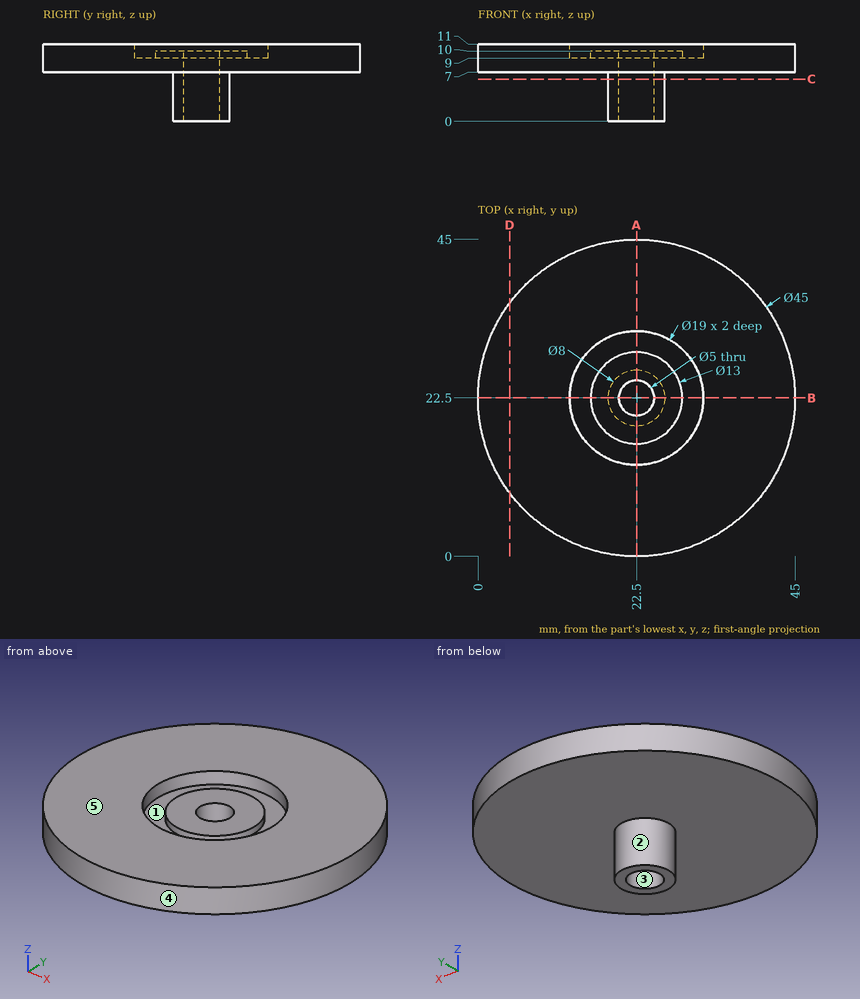
Check sheet for the drawn part. Datum: minimum x, y, z corner. Units: mm. A direction names the side the tool comes from. Give positions to 0.01 mm unless a question says otherwise; leave off trailing zeros. Order: outer loops, then holes, each group sorted by start corner. A loop starts at its lowest first (then second) coordinate and runs counter-clockwise, first axis right, second up. Notation, with made-up numbers: (5.5, 25) -> (40.5, 25) arc R22 cw to (40.5, 42) -> close; hole circle Ø4 at (-35.75, 85.25). An arc over 180 degrees is marked (long way). Use a Markdown table: item, result.
1) Mould release check, pull along X, two halves, no side actions. Record for the marked faces 3, 4 and 5: pulls with the +X half, pulls with the -X half, needs draft (parallel to the pull), parting line crosses it, or undercut.
Results:
| item | result |
|---|---|
| face 3 | undercut |
| face 4 | parting line crosses it |
| face 5 | needs draft |
2) Depth check by flat-ended pin: pin 1 Ø4 at (x, y) = (21, 24) entering from +Z; pin 2 Ø1.5 at (x, z) = (40, 7.5) entering from -Y; pin 3 Ø5 at (x, y) = (38.5, 10) entering from -Z. Enter the tip coordinate at first touch or a pass-through.
Results:
| item | result |
|---|---|
| pin 1 | z = 10 |
| pin 2 | y = 7.48 |
| pin 3 | z = 7 |
3) Material ranges on probe 1 along X at (y, z) = (22.5, 7.25); probe 2 along X at (y, z) = (22.5, 3.75); probe 3 along Z at (x, y) = (41, 15.5), recorded low to high.
Results:
| item | result |
|---|---|
| probe 1 | 0 to 20, 25 to 45 |
| probe 2 | 18.5 to 20, 25 to 26.5 |
| probe 3 | 7 to 11 |
4) Section check D-D, the plane x = 4.5. Record the boundary of the cut face in (y, z).
Results:
| item | result |
|---|---|
| outline | (9, 7) -> (36, 7) -> (36, 11) -> (9, 11) -> close |
5) Section check C-C, the plane z = 6. Record the boundary of the cut face in (x, y), then the cut area to 3 significant figures.
Results:
| item | result |
|---|---|
| outline | circle Ø8 at (22.5, 22.5); hole circle Ø5 at (22.5, 22.5) |
| area | 30.6 mm² |
6) Section check A-A, the plane x = 22.5. Record the boundary of the cut face in (y, z).
Results:
| item | result |
|---|---|
| outline | (0, 7) -> (18.5, 7) -> (18.5, 0) -> (20, 0) -> (20, 10) -> (16, 10) -> (16, 9) -> (13, 9) -> (13, 11) -> (0, 11) -> close; (25, 0) -> (26.5, 0) -> (26.5, 7) -> (45, 7) -> (45, 11) -> (32, 11) -> (32, 9) -> (29, 9) -> (29, 10) -> (25, 10) -> close |
7) Tool access check on the marked faces 1 and 2. Record the directions out of +Z, -Z, +X, -X, +Y, -Y that give a thin tool (end or side, any length) a straight path to the whole face; none if there is none.
Results:
| item | result |
|---|---|
| face 1 | +Z |
| face 2 | -Z |
